from build123d import *

# Parameters (mm, degrees)
SKETCH_W          = 4
SKETCH_H          = 20
SKETCH001_R       = 4
PAD_DEPTH         = 5
SKETCH002_R       = 1.5
POCKET_DEPTH      = 5.001
POCKET_DEPTH_BACK = -5.001
SKETCH003_R       = 2
POCKET001_DEPTH   = 15


with BuildPart() as part:
    # Sketch (on DatumPlane) → Revolution (revolve)
    with BuildSketch(Plane.XZ):
        with Locations((2, 10)):
            Rectangle(SKETCH_W, SKETCH_H)
    revolve(axis=Axis((0, 0, 0), (0, 0, 1)))

    # Sketch001 (on DatumPlane) → Pad (new body, symmetric)
    with BuildSketch(Plane.YZ):
        Circle(SKETCH001_R)
    extrude(amount=PAD_DEPTH, both=True)

    # Sketch002 (on DatumPlane) → Pocket (cut, two sides)
    with BuildSketch(Plane.YZ) as pocket_sk:
        Circle(SKETCH002_R)
    extrude(amount=-POCKET_DEPTH, mode=Mode.SUBTRACT)
    extrude(pocket_sk.sketch, amount=-POCKET_DEPTH_BACK, mode=Mode.SUBTRACT)

    # Sketch003 (on DatumPlane) → Pocket001 (cut)
    with BuildSketch(Plane.XY.offset(20)):
        Circle(SKETCH003_R)
    extrude(amount=-POCKET001_DEPTH, mode=Mode.SUBTRACT)


solid = part.part
The listing builds one solid part. Answer for the finished solid, in the listing's coordinates (mm). A direction names the side the tool comes from. Round coordinates to 2 decimals unless told otherwise and drop trailing zeros. Write each loop counter-clockwise with the first axis right and the second up, starting at its lowest first coordinate (ties: lowest second). Pieces come first, ordered by that corner, then holes. Notation, with made-up numbers: (-14, 31) - (23, 31) arc R23 cw to (23, 46) - close; hole circle Ø11 at (-8.5, 15.25). An arc over 180 degrees is marked (long way). Use one line per item in the form item = value. Start each with the question number.
Item 1: A cutting plane is placed at C-C (z = 2). Write down the section's boundary in (x, y).
Item 2: A cutting plane is placed at B-B (x = -1.75). Write down the section's boundary in (y, z), plus the area to 3 significant figures.
Item 3: Find the intervals of material crossed by line 1 (Y direction, x = 0, z = 10); line 2 (Y direction, x = 3.7, z = 0); line 3 (X direction, y = 1.75, z = 9), in increasing order. Write a range as [from, to].
Item 4: Flat-ended cylindrical pins translate along their axes: pin 1 Ø1 at (x, z) = (3, 17.5) entering from +Y; pin 2 Ø4 at (y, z) = (0, 0) entering from -X; pin 3 Ø4 at (y, z) = (0.5, 7) entering from +X; pin 4 Ø4 at (y, z) = (-2.5, 10) entering from -X. Find the tip coordinate at first contact, or state that the pin passes through.
Item 5: A cutting plane is placed at A-A (y = 0). Write down the section's boundary in (x, z), plus the area to 3 significant figures.
Item 6: A cutting plane is placed at D-D (y = 3.25). Write down the section's boundary in (x, z), plus the area to 3 significant figures.
Item 7: Determine the mould class of faces 1 (the cylindrical face through (-4, 0, 12)), 2 (the flat face through (-5, 2, 0)), 3 (the flat face through (0, 0, 5)) for opening direction X: +X half, -X half, draft (parallel to the pull), parting line (faces both ways), or undercut.
Item 8: A tool of negligible diameter and unlimited length cuts with its end or side. For faces 4 (the cylindrical face through (0.07, -0.867, -3.905)), 5 (the cylindrical face through (0, -2, 13)), 6 (the flat face through (5, 2, 0)), from which of +Z, -Z, +X, -X, +Y, -Y can it reach the whole face along a straight path? Write none if from no direction.
The answers:
q1.outline = (-5, -3.46) - (-2, -3.46) arc R4 ccw to (2, -3.46) - (5, -3.46) - (5, 3.46) - (2, 3.46) arc R4 ccw to (-2, 3.46) - (-5, 3.46) - close
q2.outline = (-3.6, 1.75) arc R4 ccw (long way) to (3.6, 1.75) - (3.6, 20) - (0.97, 20) - (0.97, 5) - (-0.97, 5) - (-0.97, 20) - (-3.6, 20) - close; hole circle Ø3 at (0, 0)
q2.area = 134 mm^2
q3.line_1 = [-4, -2], [2, 4]
q3.line_2 = [-4, -1.5], [1.5, 4]
q3.line_3 = [-3.6, -0.97], [0.97, 3.6]
q4.pin_1 = 3.12
q4.pin_2 = -5
q4.pin_3 = 4
q4.pin_4 = -3.97
q5.outline = (-5, -4) - (5, -4) - (5, -1.5) - (-5, -1.5) - close; (-5, 1.5) - (5, 1.5) - (5, 4) - (4, 4) - (4, 20) - (2, 20) - (2, 5) - (-2, 5) - (-2, 20) - (-4, 20) - (-4, 4) - (-5, 4) - close
q5.area = 118 mm^2
q6.outline = (-5, -2.33) - (5, -2.33) - (5, 2.33) - (2.33, 2.33) - (2.33, 20) - (-2.33, 20) - (-2.33, 2.33) - (-5, 2.33) - close
q6.area = 129 mm^2
q7.face_1 = parting line
q7.face_2 = -X half
q7.face_3 = undercut
q8.face_4 = none
q8.face_5 = +Z
q8.face_6 = +Z, -Z, +X, +Y, -Y
